Input: part model. Units: mm. Frame: model coordinates. A direction names the side the tool comes from. Give positions to 0.01 mm unless a question says otherwise; leave off trailing zeros. Loops run counter-clockwise (first coordinate to the right, second up) from the corner with the lowest first, then second, coordinate; pieces in that order, holes last. Notation, with made-up numbers: M 76.5,31.25 L 85.5,31.25 A23 ccw 85.5,42.25 Z; hole C 68,-40 d11. An arc over 180 degrees is marked long. One line per item, written item: value. Start each with the question number.
(1) Pull-direction query (Y, two-part tool) for faces 1 (the flat face through (-21, 20, 1)), 2 (the flat face through (-46, 5, 0)), 3 (the flat face through (-1.98, 0, 1.15)), 4 (the cylindrical face through (-50.496, 0.176, 0.986)); classes: released by +Y, released by -Y, zero draft, split by the parting line, or undercut.
(2) Access query for faces 5 (the flat face through (-4.5, 5, 1)), 6 (the flat face through (-4.5, -15, 1)), 7 (the cylindrical face through (-84.496, 0.176, 0.986)). Directions: +Z, -Z, +X, -X, +Y, -Y. A direction counts if a zero-diameter tool reaches every point of the face in a straight line with its end or side. Return the directions, or none.
(3) Section B-B on x = -19.5. Output: boundary loops of the cut face in (y, z).
(4) Ray query, line 1 along Y through (x, z) = (-19.5, 0.4); line 2 along X through (y, z) = (18.5, -2.5); line 3 along Z through (x, y) = (-61, -14). Return the intervals inside material, ascending. Write a range as from..to.
(5) Section D-D on y = -12. Output: boundary loops of the cut face in (x, z).
(6) Pin query (flat end, axial travel): P1, Ø2, axis at y = 12, z = -4, coming from the -X side; P2, Ø4, axis at x = -52.5, z = 0.5, coming from the +Y side; P3, Ø5, axis at x = -61.5, y = -6, coming from the -Z side. Return the tip coordinate at first contact, or that it passes through.
(7) Section C-C on y = 12. Output: boundary loops of the cut face in (x, z), plus the area to 3 significant figures.
(8) Section A-A on z = -2.5. Output: boundary loops of the cut face in (x, y).
```python
from build123d import *

# Parameters (mm, degrees)
BOSS_EXTRUDE1_DEPTH     = 2
SKETCH12_R              = 4.5
SKETCH12_R_2            = 4
BOSS_EXTRUDE12_DEPTH    = 20
CUT_EXTRUDE1_DEPTH      = 93.460802506
CUT_EXTRUDE1_DEPTH_BACK = 93.460802506
SKETCH3_R               = 4


with BuildPart() as part:
    # Sketch2 → Boss-Extrude1 (new body)
    with BuildSketch(Plane.XY):
        with BuildLine():
            Line((-4, 20), (-46.5, 20))
            Line((-46.5, 20), (-82.211080106, 10.211252251))
            ThreePointArc((-82.211080106, 10.211252251), (-90, 0), (-82.211080106, -10.211252251))
            Line((-82.211080106, -10.211252251), (-46.5, -20))
            Line((-46.5, -20), (-4, -20))
            Line((-4, -20), (-4, -10))
            Line((-4, -10), (-4, 0))
            Line((-4, 0), (-4, 10))
            Line((-4, 10), (-4, 20))
        make_face()
    extrude(amount=BOSS_EXTRUDE1_DEPTH)

    # Sketch12 → Boss-Extrude12 (add, symmetric)
    # profile 1 of 2: a face of its own
    with BuildSketch(Plane(origin=(0, 0, 0), x_dir=(1, 0, 0), z_dir=(0, 1, 0))):
        with Locations((0, 2.5)):
            Circle(SKETCH12_R)
        with Locations(Location((0, 2.5, 0), (0, 0, 270))):
            Circle(SKETCH12_R_2, mode=Mode.SUBTRACT)
    # profile 2 of 2: a face of its own
    with BuildSketch(Plane(origin=(0, 0, 0), x_dir=(1, 0, 0), z_dir=(0, 1, 0))):
        with BuildLine():
            Line((-4, 0), (-4, -2))
            Line((-4, -2), (0, -2))
            ThreePointArc((0, -2), (-2.121320344, -1.468626967), (-3.741657387, 0))
            Line((-3.741657387, 0), (-4, 0))
        make_face()
    extrude(amount=BOSS_EXTRUDE12_DEPTH, both=True)

    # Sketch3 → Cut-Extrude1 (cut, two sides: drawn at the far end of the back side and taken through both)
    with BuildSketch(Plane.XY.offset(-CUT_EXTRUDE1_DEPTH_BACK)):
        with Locations((-19.5, -12)):
            Circle(SKETCH3_R)
        with Locations((-19.5, 12)):
            Circle(SKETCH3_R)
        with Locations((-46.5, 0)):
            Circle(SKETCH3_R)
        with Locations((-80.5, 0)):
            Circle(SKETCH3_R)
        Polygon((0, 10), (4.5, 10), (4.5, 0), (-4.5, 0), (-4.5, 10), align=None)
        Polygon((0, -10), (4.5, -10), (4.5, -20), (0, -20), (-4.5, -20), (-4.5, -10), align=None)
    extrude(amount=CUT_EXTRUDE1_DEPTH + CUT_EXTRUDE1_DEPTH_BACK, mode=Mode.SUBTRACT)


solid = part.part
```
Output values:
1. face 1: released by +Y
1. face 2: zero draft
1. face 3: undercut
1. face 4: undercut
2. face 5: +Z, -Z, +X
2. face 6: +Z, -Z, +X, -Y
2. face 7: +Z, -Z
3. outline: M -20,0 L -16,0 L -16,2 L -20,2 Z; M -8,0 L 8,0 L 8,2 L -8,2 Z; M 16,0 L 20,0 L 20,2 L 16,2 Z
4. line 1: y = -20..-16, -8..8, 16..20
4. line 2: x = -4.5..-4, 4..4.5
4. line 3: z = 0..2
5. outline: M -75.69,0 L -23.5,0 L -23.5,2 L -75.69,2 Z; M -15.5,0 L -4.5,0 L -4.5,2 L -15.5,2 Z
6. P1: stops at x = -4.47
6. P2: stops at y = 18.9
6. P3: stops at z = 0
7. outline: M -75.69,0 L -23.5,0 L -23.5,2 L -75.69,2 Z; M -15.5,0 L -3.74,0 A4.5 ccw long 0,2 L -15.5,2 Z; hole C 0,-2.5 d8
7. area: 143 mm²
8. outline: M -4.5,-10 L -4,-10 L -4,0 L -4.5,0 Z; M -4.5,10 L -4,10 L -4,20 L -4.5,20 Z; M 4,-10 L 4.5,-10 L 4.5,0 L 4,0 Z; M 4,10 L 4.5,10 L 4.5,20 L 4,20 Z
